Solid Edge part; units mm, degrees
sketch "Sketch1" plane through (0, 0, 0) normal (0, 0, 1) x (1, 0, 0)
  line L0 (40, 0) -> (0, 0)
  line L1 (0, 0) -> (0, 30)
  line L2 (0, 30) -> (40, 30)
  arc A0 (40, 30) -> (40, 0) centre (40, 15) cw
extrude "Protrusion1" add sketch "Sketch1" along normal blind 10
sketch "Sketch2" plane through (0, 15, 5) normal (-1, 0, 0) x (0, 1, 0)
  line L0 (-15, -35) -> (-15, 5)
  line L1 (-15, 5) -> (15, 5)
  line L2 (15, 5) -> (15, -35)
  arc A0 (15, -35) -> (-15, -35) centre (0, -35) cw
  circle A1 centre (0, -35) radius 7.5
extrude "ExtrudedCutout_2" cut sketch "Sketch2" against normal blind 10
sketch "Sketch3" plane through (0, 15, 5) normal (-1, 0, 0) x (0, 1, 0)
  line L0 (-15, -35) -> (-15, 5)
  line L1 (-15, 5) -> (15, 5)
  line L2 (15, 5) -> (15, -35)
  arc A0 (15, -35) -> (-15, -35) centre (0, -35) cw
  circle A1 centre (0, -35) radius 7.5
extrude "ExtrudedProtrusion_3" add sketch "Sketch3" against normal blind 10
sketch "Sketch4" plane through (0, 15, 0) normal (0, -1, 0) x (1, 0, 0)
  line L0 (40, 10) -> (10, 30)
  line L1 (10, 10) -> (10, 30)
  line L2 (10, 10) -> (40, 10)
extrude "ExtrudedProtrusion_8" add sketch "Sketch4" along normal mid plane 10
Work out the finished part from the listing and answer in its coordinate system (mm). A direction names the side the tool comes from. Give positions to 0.01 mm unless a question says otherwise; leave off trailing zeros. Write each loop counter-clockwise with the first axis right and the second up, starting at its lowest first coordinate (ties: lowest second). Pieces come first, ordered by that corner, then holes. Notation, with made-up numbers: M 43.25,-25 L 90.25,-25 A25 cw 90.25,-3 Z; hole C 10,23 d8. An arc over 180 degrees is marked long. Answer as CSV lines item,"result".
Q1. A cutting plane is placed at A-A on y = 15. Write down the section's boundary in (x, z).
A:
outline,"M 0,0 L 55,0 L 55,10 L 40,10 L 10,30 L 10,32.5 L 0,32.5 Z; M 0,47.5 L 10,47.5 L 10,55 L 0,55 Z"
Q2. The mould has two halves that part along Y. Classify faces 1 (the cylindrical face through (4.93, 13.37, 47.32)), 2 (the flat face through (28, 15, 0)), 3 (the flat face through (19, 20, 16)): +Y half, -Y half, draft (parallel to the pull), parting line (faces both ways), or undercut.
A:
face 1,"undercut"
face 2,"draft"
face 3,"+Y half"
Q3. Given P1, Ø22, axis at x = 22.5, z = 23, coming from the +Y side; P2, Ø8, axis at x = 39.5, z = 15, coming from the -Y side; P3, Ø4, axis at y = 16.5, z = 19, coming from the +X side; P4, Ø12, axis at y = 15, z = 40, coming from the -X side, each flat-ended and moving along its own axis, determine where each tip first touches the part or whether it passes through.
A:
P1,"stops at y = 20"
P2,"stops at y = 10"
P3,"stops at x = 29.5"
P4,"passes through"
Q4. A cutting plane is placed at D-D on z = 26. Write down the section's boundary in (x, y).
A:
outline,"M 0,0 L 10,0 L 10,10 L 16,10 L 16,20 L 10,20 L 10,30 L 0,30 Z"
Q5. A tool of negligible diameter and unlimited length cuts with its end or side. For faces 4 (the flat face through (25, 15, 20)), 5 (the flat face through (10, 15, 32)), 6 (the flat face through (19, 10, 16)), from which of +Z, -Z, +X, -X, +Y, -Y can it reach the whole face along a straight path? Write none if from no direction.
A:
face 4,"+Z, +X, +Y, -Y"
face 5,"+Z, +X"
face 6,"+Z, +X, -Y"
Q6. A cutting plane is placed at C-C on z = 44.5. Write down the section's boundary in (x, y).
A:
outline,"M 0,0.69 L 10,0.69 L 10,9 L 0,9 Z; M 0,21 L 10,21 L 10,29.31 L 0,29.31 Z"
Q7. A cutting plane is placed at B-B on x = 32.5. Write down the section's boundary in (y, z).
A:
outline,"M 0,0 L 30,0 L 30,10 L 20,10 L 20,15 L 10,15 L 10,10 L 0,10 Z"
Q8. Find the intervals of material crossed by probe 1 along Z at (x, y) = (3, 15); probe 2 along Y at (x, z) = (7.25, 40); probe 3 along Z at (x, y) = (42, 12.75), in increasing order. Write a range as [from, to].
A:
probe 1,"z = [0, 32.5], [47.5, 55]"
probe 2,"y = [0, 7.5], [22.5, 30]"
probe 3,"z = [0, 10]"
